from build123d import *
from build123d.topology import SkipClean

# Parameters (mm, degrees)
SKETCH_2_R                   = 25
SKETCH_2_R_2                 = 10
EXTRUDE_2_DEPTH              = 2
SKETCH_35_R                  = 13.5
EXTRUDE_3_DEPTH              = 2
SKETCH_36_R                  = 12.5
EXTRUDE_4_DEPTH              = 7
HOLE_WIZARD_M3_1_D           = 3.4
HOLE_WIZARD_M3_1_CBORE_D     = 6.5
HOLE_WIZARD_M3_1_CBORE_DEPTH = 3.4
PATTERN_CIRCULAR_1_COUNT     = 3
PATTERN_CIRCULAR_2_COUNT     = 3
EXTRUDE_START                = 3
SKETCH_53_R                  = 11.5
SKETCH_53_R_2                = 1.65
SKETCH_53_R_3                = 3.25
EXTRUDE_5_DEPTH              = 3
EXTRUDE_START_2              = 7
SKETCH_61_R                  = 10
SKETCH_61_R_2                = 1.7
EXTRUDE_6_DEPTH              = 7
SKETCH_62_R                  = 10
SKETCH_62_R_2                = 9.5
CUT_EXTRUDE_1_DEPTH          = 5
FILLET_1_R                   = 0.1
PATTERN_CIRCULAR_3_COUNT     = 3
PATTERN_CIRCULAR_4_COUNT     = 2


with BuildPart() as part:
    # 스케치2 → 보스-돌출2 (new body)
    with BuildSketch(Plane(origin=(0, 6, 0), x_dir=(1, 0, 0), z_dir=(0, 0, -1))):
        with Locations(Location((0, 6, 0), (0, 0, 180))):
            Circle(SKETCH_2_R)
        with Locations(Location((0, 6, 0), (0, 0, 180))):
            Circle(SKETCH_2_R_2, mode=Mode.SUBTRACT)
    extrude(amount=EXTRUDE_2_DEPTH)

    # 스케치35 → 보스-돌출3 (add)
    with BuildSketch(Plane(origin=(0, 0, -2), x_dir=(-1, 0, 0), z_dir=(0, 0, -1))):
        Circle(SKETCH_35_R)
    extrude(amount=EXTRUDE_3_DEPTH)

    # 스케치36 → 보스-돌출4 (add)
    with BuildSketch(Plane(origin=(0, 0, -4), x_dir=(-1, 0, 0), z_dir=(0, 0, -1))):
        Circle(SKETCH_36_R)
    extrude(amount=EXTRUDE_4_DEPTH)

    # M3 육각 소켓 머리 캡 나사용 카운터보어1 (through all)
    with Locations(Plane(origin=(0, 0, -11), x_dir=(-1, 0, 0), z_dir=(0, 0, -1))):
        with Locations((0, 4)):
            hole_wizard_m3_1 = CounterBoreHole(HOLE_WIZARD_M3_1_D / 2, HOLE_WIZARD_M3_1_CBORE_D / 2, HOLE_WIZARD_M3_1_CBORE_DEPTH)

    # 원형 패턴1: M3 육각 소켓 머리 캡 나사용 카운터보어1 ×3 about axis
    pattern_circular_1_axis = Axis((0, 0, 0), (0, 0, 1))
    for i in range(1, PATTERN_CIRCULAR_1_COUNT):
        add(hole_wizard_m3_1.rotate(pattern_circular_1_axis, i * 360 / PATTERN_CIRCULAR_1_COUNT), mode=Mode.SUBTRACT)

    # 스케치52 → M4 탭을 위한 탭 드릴1 (revolve, cut)
    with BuildSketch(Plane(origin=(0, -7, -11), x_dir=(0, 1, 0), z_dir=(1, 0, 0))):
        Polygon((0, 0), (0, 5.991420021), (1.65, 5), (1.65, 0), align=None)
    hole_wizard_m4_1 = revolve(axis=Axis((0, -7, -17.35), (0, 0, 1)), mode=Mode.SUBTRACT)

    # 원형 패턴2: M4 탭을 위한 탭 드릴1 ×3 about axis
    pattern_circular_2_axis = Axis((0, 0, 0), (0, 0, 1))
    for i in range(1, PATTERN_CIRCULAR_2_COUNT):
        add(hole_wizard_m4_1.rotate(pattern_circular_2_axis, i * 360 / PATTERN_CIRCULAR_2_COUNT), mode=Mode.SUBTRACT)

    # 스케치53 → 보스-돌출5 (add)
    with SkipClean():  # the faces are left unmerged after this step: merging them gives an invalid solid
        with BuildSketch(Plane(origin=(0, 0, -11), x_dir=(-1, 0, 0), z_dir=(0, 0, -1)).offset(EXTRUDE_START)):
            Circle(SKETCH_53_R)
            with Locations((6.062177826, 3.5)):
                Circle(SKETCH_53_R_2, mode=Mode.SUBTRACT)
            with Locations((0, -7)):
                Circle(SKETCH_53_R_2, mode=Mode.SUBTRACT)
            with Locations((3.464101615, -2)):
                Circle(SKETCH_53_R_3, mode=Mode.SUBTRACT)
            with Locations((0, 4)):
                Circle(SKETCH_53_R_3, mode=Mode.SUBTRACT)
            with Locations((-3.464101615, -2)):
                Circle(SKETCH_53_R_3, mode=Mode.SUBTRACT)
            with Locations((-6.062177826, 3.5)):
                Circle(SKETCH_53_R_2, mode=Mode.SUBTRACT)
        extrude(amount=-EXTRUDE_5_DEPTH)

    # 스케치61 → 보스-돌출6 (add)
    with BuildSketch(Plane.XY.offset(-2).offset(EXTRUDE_START_2)):
        with Locations(Location((0, 0, 0), (0, 0, 180))):
            Circle(SKETCH_61_R)
        with Locations(Location((-3.464101615, -2, 0), (0, 0, 180))):
            Circle(SKETCH_61_R_2, mode=Mode.SUBTRACT)
        with Locations(Location((3.464101615, -2, 0), (0, 0, 180))):
            Circle(SKETCH_61_R_2, mode=Mode.SUBTRACT)
        with Locations(Location((0, 4, 0), (0, 0, 180))):
            Circle(SKETCH_61_R_2, mode=Mode.SUBTRACT)
    extrude(amount=-EXTRUDE_6_DEPTH)

    # 스케치62 → 컷-돌출1 (cut)
    with BuildSketch(Plane.XY.offset(5)):
        Circle(SKETCH_62_R)
        Circle(SKETCH_62_R_2, mode=Mode.SUBTRACT)
    extrude(amount=-CUT_EXTRUDE_1_DEPTH, mode=Mode.SUBTRACT)

    # 필렛1
    fillet_1_edges = [part.edges().sort_by_distance(p)[0] for p in [
        (-9.5, 0, 0),
        (-9.5, 0, 5),
    ]]
    fillet(fillet_1_edges, radius=FILLET_1_R)

    # 스케치67 → Ø3.0mm 맞춤핀 구멍1 (revolve, cut)
    with BuildSketch(Plane(origin=(0, -7, 5), x_dir=(0, -1, 0), z_dir=(1, 0, 0))):
        Polygon((0, 0), (0, 5.901290929), (1.5, 5), (1.5, 0), align=None)
    f_3_0mm_1 = revolve(axis=Axis((0, -7, 11.35), (0, 0, -1)), mode=Mode.SUBTRACT)

    # 원형 패턴3: Ø3.0mm 맞춤핀 구멍1 ×3 about axis
    pattern_circular_3_axis = Axis((0, 0, 0), (0, 0, 1))
    for i in range(1, PATTERN_CIRCULAR_3_COUNT):
        add(f_3_0mm_1.rotate(pattern_circular_3_axis, i * 360 / PATTERN_CIRCULAR_3_COUNT), mode=Mode.SUBTRACT)

    # 스케치79 → Ø3.0mm 맞춤핀 구멍4 (revolve, cut)
    with BuildSketch(Plane(origin=(-4.25, 7.361215932, -14), x_dir=(0, 1, 0), z_dir=(1, 0, 0))):
        Polygon((0, 0), (0, 5.901290929), (1.5, 5), (1.5, 0), align=None)
    f_3_0mm_4 = revolve(axis=Axis((-4.25, 7.361215932, -20.35), (0, 0, 1)), mode=Mode.SUBTRACT)

    # 원형 패턴4: Ø3.0mm 맞춤핀 구멍4 ×2 about axis
    pattern_circular_4_axis = Axis((0, 0, 0), (0, 0, 1))
    for i in range(1, PATTERN_CIRCULAR_4_COUNT):
        add(f_3_0mm_4.rotate(pattern_circular_4_axis, i * 360 / PATTERN_CIRCULAR_4_COUNT), mode=Mode.SUBTRACT)


solid = part.part
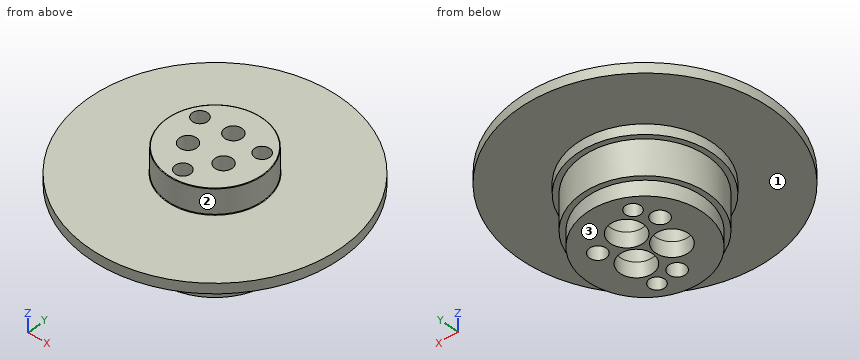
Part model, mm, in its own coordinate system. Face numbers are marked on the shaded views. A direction names the side the tool comes from. Give positions to 0.01 mm unless a question says otherwise; leave off trailing zeros. Loops run counter-clockwise (first coordinate to the right, second up) from the corner with the lowest first, then second, coordinate; pieces in that order, holes last. Notation, with made-up numbers: M 2,63 L 36,63 A24 ccw 36,86 Z; hole C 59.25,30 d8. An arc over 180 degrees is marked long. Put each result on its own line as item: value. Start each with the question number.
1) Probe probe 1 along Y at (x, z) = (0, 1.6); probe 2 along Y at (x, z) = (0, -11.5); probe 3 along X at (y, z) = (3.5, -12.3). List the from-to ranges inside material, lowest first.
2) Saw through at C-C (x = -10.5). List the corners of the cut face in (y, z).
3) Saw through at D-D (x = 14.5). List the corners of the cut face in (y, z).
4) 3-axis set-ups, long thin cutter, end or side, ignore diameter. For the marked faces 1, 2 and 3: which of +Z, -Z, +X, -X, +Y, -Y reach the whole face in a straight line?
5) Saw through at A-A (z = 2). List the corners of the cut face in (x, y).
6) Flat gauge pins, fed straight in: pin 1 (5 mm diameter, centred on x = -3, z = -11.5, fed in from -Y); pin 2 (2 mm diameter, centred on y = -7.5, z = -8.5, fed in from +X); pin 3 (2 mm diameter, centred on x = 0, y = -7, fed in from -Z); pin 4 (2.5 mm diameter, centred on x = -3.46, y = -2, fed in from +Z). Where does each tip first touch, or does it go through?
7) Saw through at B-B (y = 20). List the corners of the cut face in (x, z).
Numbers:
1. probe 1: -9.5 to -8.5, -5.5 to 2.3, 5.7 to 9.5
1. probe 2: -11.5 to -8.65, -5.35 to 0.75, 7.25 to 11.5
1. probe 3: -10.95 to -7.71, -4.41 to -3.21, 3.21 to 4.41, 7.71 to 10.95
2. outline: M -22.69,-2 L -8.49,-2 L -8.49,-4 L -6.78,-4 L -6.78,-11 L -4.69,-11 L -4.69,-14 L 4.69,-14 L 4.69,-11 L 6.78,-11 L 6.78,-4 L 8.49,-4 L 8.49,-2 L 22.69,-2 L 22.69,0 L -22.69,0 Z
3. outline: M -20.37,-2 L 20.37,-2 L 20.37,0 L -20.37,0 Z
4. face 1: -Z
4. face 2: +Z
4. face 3: -Z, +X, -X, +Y, -Y
5. outline: C 0,0 d19; hole C -6.06,3.5 d3; hole C -3.46,-2 d3.4; hole C 0,4 d3.4; hole C 0,-7 d3; hole C 3.46,-2 d3.4; hole C 6.06,3.5 d3
6. pin 1: y = -12.49
6. pin 2: x = 10.68
6. pin 3: z = -5.61
6. pin 4: through
7. outline: M -15,-2 L 15,-2 L 15,0 L -15,0 Z
